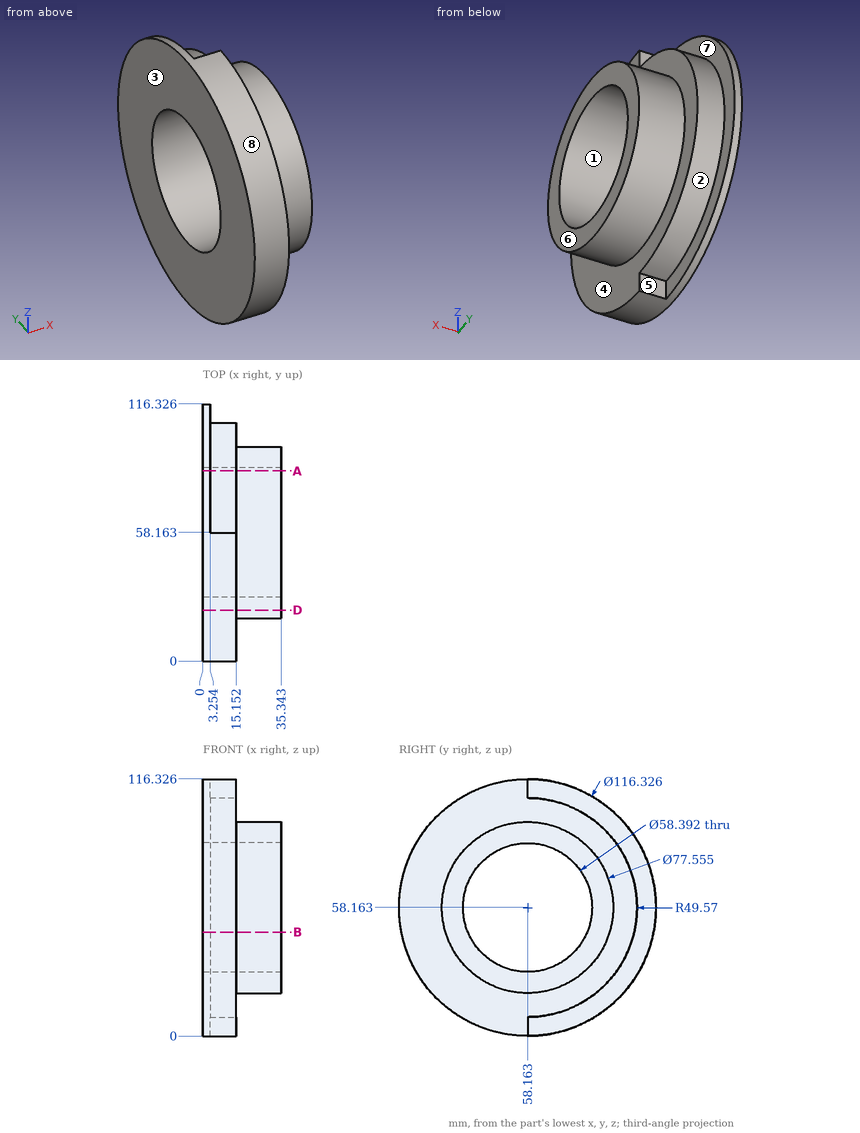
Geometry: see drawing. Coordinates: mm, zero at the bounding-box minimum. A direction names the side the tool comes from. Give positions to 0.01 mm unless a question says otherwise; leave off trailing zeros. Write each loop counter-clockwise with the first axis right and the second up, starting at its lowest first coordinate (ties: lowest second). Pieces come first, ordered by that corner, then holes. Notation, with made-up numbers: (75, -18.75) - (103, -18.75) arc R19 cw to (103, -0.75) - close; hole circle Ø8 at (13, -32.5). An arc over 180 degrees is marked (long way). Return JSON: item names as keys, results as strings. Group by question number.
1) Mould query, pull axis Z, two halves, no side actions, for the marked faces 1, 2 and 3. Classes: released by +Z, released by -Z, zero draft, split by the parting line, or undercut.
2) Section B-B on z = 47. Return the cut outline in (x, y) (1 decimal).
3) Set-up query: the marked faces 4, 5, 6, 7 and 8. Return all of +Z, -Z, +X, -X, +Y, -Y with unobstructed straight access to the full face (end or side cutting, diameter ignored); none if empty.
4) Section D-D on y = 23. Return the cut outline in (x, z) (1 decimal).
5) Section A-A on y = 86. Return the cut outline in (x, z) (1 decimal).
6) Line query: line 1 (X direction, y = 87.5, z = 89); line 2 (Z direction, x = 19, y = 57.5) (1 decimal); line 3 (Y direction, x = 17, z = 40.5) (1 decimal). Output: solid intervals per line, ascending.
7) First-contact query: P1, Ø2, axis at x = 6, y = 84, coming from the +Z side; P2, Ø1, axis at x = 18.5, z = 57.5, coming from the +Y side; P3, Ø2, axis at x = 19.5, y = 32.5, coming from the -Z side. Flat tips, straight axial feed; report the tip coordinate or a pass-through.
Filled in:
{
 "1": {"face 1": "undercut", "face 2": "split by the parting line", "face 3": "zero draft"},
 "2": {"outline": "(0, 1.1) - (15.2, 1.1) - (15.2, 21) - (35.3, 21) - (35.3, 31.2) - (0, 31.2) - close; (0, 85.1) - (35.3, 85.1) - (35.3, 95.3) - (15.2, 95.3) - (15.2, 106.5) - (3.3, 106.5) - (3.3, 115.2) - (0, 115.2) - close"},
 "3": {"face 4": "+X", "face 5": "-Z, +X, +Y", "face 6": "+Z, -Z, +X, +Y, -Y", "face 7": "+X, +Y", "face 8": "+X, -X"},
 "4": {"outline": "(0, 11.8) - (15.2, 11.8) - (15.2, 41.8) - (35.3, 41.8) - (35.3, 74.5) - (15.2, 74.5) - (15.2, 104.5) - (0, 104.5) - close"},
 "5": {"outline": "(0, 7.1) - (3.3, 7.1) - (3.3, 17.1) - (15.2, 17.1) - (15.2, 31.2) - (35.3, 31.2) - (35.3, 49.4) - (0, 49.4) - close; (0, 67) - (35.3, 67) - (35.3, 85.2) - (15.2, 85.2) - (15.2, 99.2) - (3.3, 99.2) - (3.3, 109.2) - (0, 109.2) - close"},
 "6": {"line 1": "x = 0 to 15.15", "line 2": "z = 19.4 to 29, 87.4 to 96.9", "line 3": "y = 23.6 to 34.9, 81.4 to 92.7"},
 "7": {"P1": "stops at z = 101.06", "P2": "stops at y = 96.94", "P3": "stops at z = 28.24"}
}
